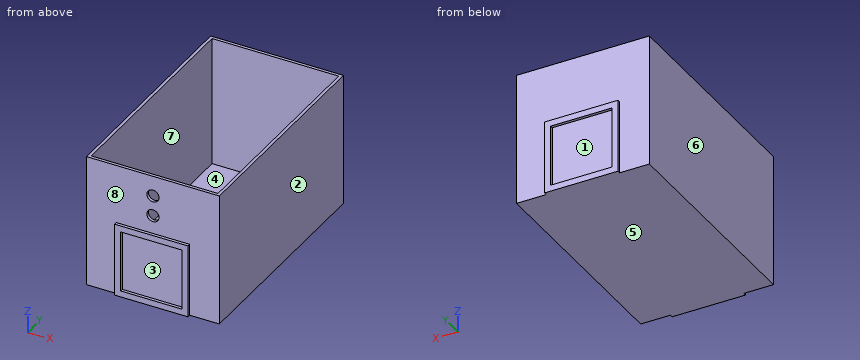
```python
from build123d import *

# Parameters (mm, degrees)
F0_W         = 65
F0_H         = 65
F1_DEPTH     = 55
F2_W         = 36
F2_H         = 36
F2_W_2       = 30
F2_H_2       = 30
F3_DEPTH     = 1.5
F5_T         = 1.5
F5_T3_DEPTH  = 39
F5_T5_DEPTH  = 39
F5_T7_DEPTH  = 4.5
F5_T9_DEPTH  = 33
F5_T11_DEPTH = 33
F5_T13_DEPTH = 4.5
F6_R         = 3
F7_DEPTH     = 1.5


# Not quite as in the source:
# - a shell that OpenCascade refuses in one call is made with other operations: the cavity is built on its own and cut out


with BuildPart() as f1:
    # F0 (on Front) → F1 (new body)
    with BuildSketch(Plane.XZ):
        with Locations((0, 32.5)):
            Rectangle(F0_W, F0_H)
    extrude(amount=F1_DEPTH)

    # F2 (on face) → F3 (join)
    with BuildSketch(Plane.XZ.offset(55)):
        with Locations((0, 18)):
            Rectangle(F2_W, F2_H)
        with Locations((0, 18)):
            Rectangle(F2_W_2, F2_H_2, mode=Mode.SUBTRACT)
    extrude(amount=F3_DEPTH)

    # F4: F1 across plane


with BuildPart() as f1_1:
    add(f1.part)
    add(f1.part.mirror(Plane.XZ))

    # F5: shell of thickness 1.5, made by hand


with BuildPart() as f5_core1:
    # F5_t2: copy of F1
    add(f1_1.part)

    # the walls: a layer under each face that stays
    f5_faces = [f5_core1.faces().sort_by_distance(p)[0] for p in [
        (-21.6666666667, 55, 10.8333333333),
        (-18, 55.75, 18),
        (-15.4285714286, 56.5, 2.5714285714),
        (0, 55.75, 3),
        (0, 55, 18),
        (15, 55.75, 18),
        (0, 55.75, 33),
        (-15, 55.75, 18),
        (0, 55.75, 36),
        (18, 55.75, 18),
        (0, 0, 0),
        (18, -55.75, 18),
        (0, -55.75, 36),
        (-15.4285714286, -56.5, 2.5714285714),
        (0, -55.75, 3),
        (0, -55, 18),
        (15, -55.75, 18),
        (0, -55.75, 33),
        (-15, -55.75, 18),
        (-18, -55.75, 18),
        (-32.5, 0, 32.5),
        (-21.6666666667, -55, 10.8333333333),
        (32.5, 0, 32.5),
    ]]
    thicken(f5_faces, amount=-F5_T, mode=Mode.SUBTRACT)

    # F5_s4 → F5_t3 (cut)
    with BuildSketch(Plane.XY.offset(-1.5)):
        Polygon((18.015, 55.015), (18, 53.5), (16.5, 53.5), (16.5, 55), align=None)
        Polygon((-18.015, 55.015), (-18, 53.5), (-16.5, 53.5), (-16.5, 55), align=None)
        Polygon((18.015, -55.015), (16.5, -55), (16.5, -53.5), (18, -53.5), align=None)
        Polygon((-18.015, -55.015), (-16.5, -55), (-16.5, -53.5), (-18, -53.5), align=None)
    extrude(amount=F5_T3_DEPTH, mode=Mode.SUBTRACT)

    # F5_s6 → F5_t5 (cut)
    with BuildSketch(Plane.YZ.offset(-19.5)):
        Polygon((55.015, 36.015), (53.5, 36), (53.5, 34.5), (55, 34.5), align=None)
        Polygon((-55.015, 36.015), (-55, 34.5), (-53.5, 34.5), (-53.5, 36), align=None)
    extrude(amount=F5_T5_DEPTH, mode=Mode.SUBTRACT)

    # F5_s8 → F5_t7 (cut)
    with BuildSketch(Plane.XZ.offset(-58)):
        Polygon((14.985, 3.015), (15, 1.5), (16.5, 1.5), (16.5, 3), align=None)
        Polygon((-14.985, 3.015), (-15, 1.5), (-16.5, 1.5), (-16.5, 3), align=None)
        Polygon((14.985, 32.985), (16.5, 33), (16.5, 34.5), (15, 34.5), align=None)
        Polygon((-14.985, 32.985), (-15, 34.5), (-16.5, 34.5), (-16.5, 33), align=None)
    extrude(amount=F5_T7_DEPTH, mode=Mode.SUBTRACT)

    # F5_s10 → F5_t9 (cut)
    with BuildSketch(Plane.YZ.offset(-16.5)):
        Polygon((55.015, 3.015), (55, 1.5), (53.5, 1.5), (53.5, 3), align=None)
        Polygon((55.015, 32.985), (53.5, 33), (53.5, 34.5), (55, 34.5), align=None)
        Polygon((-55.015, 3.015), (-55, 1.5), (-53.5, 1.5), (-53.5, 3), align=None)
        Polygon((-55.015, 32.985), (-53.5, 33), (-53.5, 34.5), (-55, 34.5), align=None)
    extrude(amount=F5_T9_DEPTH, mode=Mode.SUBTRACT)

    # F5_s12 → F5_t11 (cut)
    with BuildSketch(Plane.XY.offset(1.5)):
        Polygon((-14.985, 55.015), (-15, 53.5), (-16.5, 53.5), (-16.5, 55), align=None)
        Polygon((14.985, 55.015), (15, 53.5), (16.5, 53.5), (16.5, 55), align=None)
        Polygon((-14.985, -55.015), (-15, -53.5), (-16.5, -53.5), (-16.5, -55), align=None)
        Polygon((14.985, -55.015), (15, -53.5), (16.5, -53.5), (16.5, -55), align=None)
    extrude(amount=F5_T11_DEPTH, mode=Mode.SUBTRACT)

    # F5_s14 → F5_t13 (cut)
    with BuildSketch(Plane.XZ.offset(53.5)):
        Polygon((14.985, 3.015), (15, 1.5), (16.5, 1.5), (16.5, 3), align=None)
        Polygon((-14.985, 3.015), (-15, 1.5), (-16.5, 1.5), (-16.5, 3), align=None)
        Polygon((14.985, 32.985), (16.5, 33), (16.5, 34.5), (15, 34.5), align=None)
        Polygon((-14.985, 32.985), (-15, 34.5), (-16.5, 34.5), (-16.5, 33), align=None)
    extrude(amount=F5_T13_DEPTH, mode=Mode.SUBTRACT)


with BuildPart() as f1_2:
    add(f1_1.part)

    # what is left inside the walls is the cavity
    f5_cavity = [f5_core1.part.solids().sort_by_distance(p)[0] for p in [
        (-30.985, -17.833333, 33.25),
    ]]
    add(f5_cavity, mode=Mode.SUBTRACT)

    # F6 (on face) → F7 (cut, through all)
    with BuildSketch(Plane.XZ.offset(55)):
        with Locations((0, 55)):
            Circle(F6_R)
        with Locations((0, 45)):
            Circle(F6_R)
    extrude(amount=-F7_DEPTH, mode=Mode.SUBTRACT)


solid = f1_2.part
```
Build history of the part. All positions in model axes, mm. Face numbers are marked on the shaded views. A direction names the side the tool comes from. Round coordinates to 2 decimals unless told otherwise and drop trailing zeros. Order: outer loops, then holes, each group sorted by start corner. A loop starts at its lowest first (then second) coordinate and runs counter-clockwise, first axis right, second up. Notation, with made-up numbers: (-0.75, 72.25) -> (15.25, 72.25) arc R22 ccw to (15.25, 103.25) -> close; hole circle Ø7 at (48.5, 4.5). An arc over 180 degrees is marked (long way). Answer in a Markdown table with one row per item.
1) Band-saw the part on A-A on x = 0. Give the cut face in (y, z).
Values:
| item | result |
|---|---|
| outline | (-56.5, 0) -> (56.5, 0) -> (56.5, 3) -> (55, 3) -> (55, 33) -> (56.5, 33) -> (56.5, 36) -> (55, 36) -> (55, 65) -> (53.5, 65) -> (53.5, 1.5) -> (-53.5, 1.5) -> (-53.5, 42) -> (-55, 42) -> (-55, 36) -> (-56.5, 36) -> (-56.5, 33) -> (-55, 33) -> (-55, 3) -> (-56.5, 3) -> close; (-55, 48) -> (-53.5, 48) -> (-53.5, 52) -> (-55, 52) -> close; (-55, 58) -> (-53.5, 58) -> (-53.5, 65) -> (-55, 65) -> close |
2) Band-saw the part on B-B on z = 45. Give the cut face in (x, y).
Values:
| item | result |
|---|---|
| outline | (-32.5, -55) -> (-3, -55) -> (-3, -53.5) -> (-31, -53.5) -> (-31, 53.5) -> (31, 53.5) -> (31, -53.5) -> (3, -53.5) -> (3, -55) -> (32.5, -55) -> (32.5, 55) -> (-32.5, 55) -> close |
3) Which spindle directions (+Z, -Z, +X, -X, +Y, -Y) get a long thin tool onto all of the face, cutting with end or side? Do the marked faces 1, 2, 3, 4 and 5. Say none if no direction does.
Values:
| item | result |
|---|---|
| face 1 | +Y |
| face 2 | +Z, -Z, +X, +Y, -Y |
| face 3 | -Y |
| face 4 | +Z |
| face 5 | -Z, +X, -X, +Y, -Y |
4) Wall check: L1, parallel to Z at x = 0, y = -54.6; L2, parallel to Y at x = -4.5, z = 9.5; L3, parallel to X at y = -34.5, z = 20. Give the ranges that are in metal, low to high.
Values:
| item | result |
|---|---|
| L1 | 0 to 42, 48 to 52, 58 to 65 |
| L2 | -55 to -53.5, 53.5 to 55 |
| L3 | -32.5 to -31, 31 to 32.5 |
5) Band-saw the part on D-D on y = 32. Give the cut face in (x, z), and give its area (3 significant figures).
Values:
| item | result |
|---|---|
| outline | (-32.5, 0) -> (32.5, 0) -> (32.5, 65) -> (31, 65) -> (31, 1.5) -> (-31, 1.5) -> (-31, 65) -> (-32.5, 65) -> close |
| area | 288 mm2 |
6) Mould opens along X. For the marked faces 6, 7 and 8 say: released by +X, released by -X, zero draft, split by the parting line, or undercut.
Values:
| item | result |
|---|---|
| face 6 | released by -X |
| face 7 | undercut |
| face 8 | zero draft |
7) Pin check, flat tips, straight feed: P1, Ø1.2, axis at x = -5, y = 56, coming from the +Z side; P2, Ø1.2, axis at y = 56, z = 21.5, coming from the -X side; P3, Ø7, axis at x = 0, z = 45, coming from the -Y side. Stop position of each tip, or through.
Values:
| item | result |
|---|---|
| P1 | z = 36 |
| P2 | x = -18 |
| P3 | y = -55 |
8) Band-saw the part on C-C on x = 12.5. Give the cut face in (y, z).
Values:
| item | result |
|---|---|
| outline | (-56.5, 0) -> (56.5, 0) -> (56.5, 3) -> (55, 3) -> (55, 33) -> (56.5, 33) -> (56.5, 36) -> (55, 36) -> (55, 65) -> (53.5, 65) -> (53.5, 1.5) -> (-53.5, 1.5) -> (-53.5, 65) -> (-55, 65) -> (-55, 36) -> (-56.5, 36) -> (-56.5, 33) -> (-55, 33) -> (-55, 3) -> (-56.5, 3) -> close |
